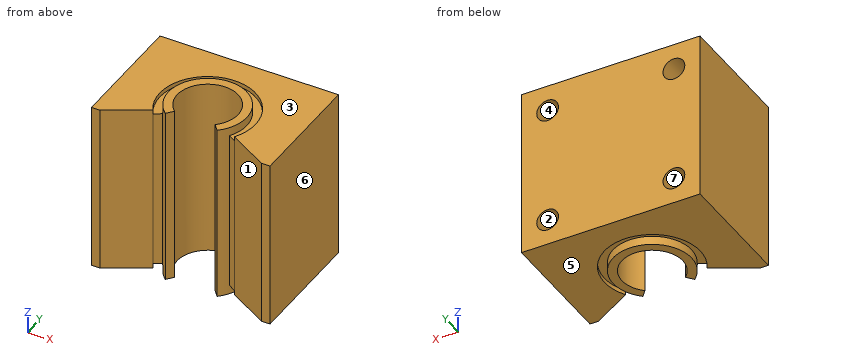
from build123d import *

# Parameters (mm, degrees)
BOSS_EXTRUDE1_DEPTH                  = 39
BOSS_EXTRUDE3_START                  = 1
BOSS_EXTRUDE3_DEPTH                  = 37
BOSS_EXTRUDE4_START                  = -1
BOSS_EXTRUDE4_DEPTH                  = 41
SKETCH4_R                            = 2.5
CUT_EXTRUDE1_DEPTH                   = 10
TAP_DRILL_FOR_M5X0_8_TAP1_AT_2_COUNT = 2
TAP_DRILL_FOR_M5X0_8_TAP1_AT_2_PITCH = 27
TAP_DRILL_FOR_M5X0_8_TAP1_AT_3_COUNT = 2
TAP_DRILL_FOR_M5X0_8_TAP1_AT_3_PITCH = 39.623223611
TAP_DRILL_FOR_M5X0_8_TAP1_AT_4_COUNT = 2
TAP_DRILL_FOR_M5X0_8_TAP1_AT_4_PITCH = 28.999998701


with BuildPart() as part:
    # Sketch1 → Boss-Extrude1 (new body)
    with BuildSketch(Plane.XY):
        with BuildLine():
            Line((-20.5, 14), (20.5, 14))
            Line((20.5, 14), (20.5, -14))
            Line((20.5, -14), (18.5, -14))
            Line((18.5, -14), (9.385134519, -8.737529961))
            ThreePointArc((9.385134519, -8.737529961), (0, 8), (-9.385134519, -8.737529961))
            Line((-9.385134519, -8.737529961), (-18.5, -14))
            Line((-18.5, -14), (-20.5, -14))
            Line((-20.5, -14), (-20.5, 14))
        make_face()
    extrude(amount=BOSS_EXTRUDE1_DEPTH)



with BuildPart() as body_2:
    # Sketch2 → Boss-Extrude3 (new body)
    with BuildSketch(Plane.XY.offset(BOSS_EXTRUDE3_START)):
        with BuildLine():
            Line((-9.385134519, -8.737529961), (-7.678746425, -7.694342695))
            ThreePointArc((-7.678746425, -7.694342695), (0, 6), (7.678746425, -7.694342695))
            Line((7.678746425, -7.694342695), (9.385134519, -8.737529961))
            ThreePointArc((9.385134519, -8.737529961), (0, 8), (-9.385134519, -8.737529961))
        make_face()
    extrude(amount=BOSS_EXTRUDE3_DEPTH)


with BuildPart() as part_1:
    add(part.part)

    add(body_2.part)  # Boss-Extrude4 merges body 2
    # Sketch3 → Boss-Extrude4 (add)
    with BuildSketch(Plane.XY.offset(BOSS_EXTRUDE4_START)):
        with BuildLine():
            Line((-5.9419479, -9.759678628), (-4.655936286, -8.227069666))
            ThreePointArc((-4.655936286, -8.227069666), (0, 4), (4.655936286, -8.227069666))
            Line((4.655936286, -8.227069666), (5.9419479, -9.759678628))
            ThreePointArc((5.9419479, -9.759678628), (0, 6), (-5.9419479, -9.759678628))
        make_face()
    extrude(amount=BOSS_EXTRUDE4_DEPTH)

    # Sketch4 → Cut-Extrude1 (cut)
    with BuildSketch(Plane(origin=(0, 14, 0), x_dir=(1, 0, 0), z_dir=(0, 1, 0))):
        with Locations(Location((-14.5, -6, 0), (0, 0, 270))):
            Circle(SKETCH4_R)
        with Locations(Location((14.499998701, -6, 0), (0, 0, 270))):
            Circle(SKETCH4_R)
        with Locations(Location((14.5, -33, 0), (0, 0, 270))):
            Circle(SKETCH4_R)
        with Locations(Location((-14.499998701, -33, 0), (0, 0, 270))):
            Circle(SKETCH4_R)
    extrude(amount=-CUT_EXTRUDE1_DEPTH, mode=Mode.SUBTRACT)

    # Sketch8 → Tap Drill for M5x0.8 Tap1 (revolve, cut)
    with BuildSketch(Plane(origin=(-14.499998701, 4, 33), x_dir=(0, 0, 1), z_dir=(1, 0, 0))):
        Polygon((0, 0), (0, 1.3118073), (2.1, 0.05), (2.1, 0.025), (2.125, 0), align=None)
    tap_drill_for_m5x0_8_tap1 = revolve(axis=Axis((-14.499998701, 10.35, 33), (0, -1, 0)), mode=Mode.SUBTRACT)

    # Tap Drill for M5x0.8 Tap1 at 2: Tap Drill for M5x0.8 Tap1 ×2
    with Locations(*[(0, 0, -i * TAP_DRILL_FOR_M5X0_8_TAP1_AT_2_PITCH) for i in range(1, TAP_DRILL_FOR_M5X0_8_TAP1_AT_2_COUNT)]):
        add(tap_drill_for_m5x0_8_tap1, mode=Mode.SUBTRACT)

    # Tap Drill for M5x0.8 Tap1 at 3: Tap Drill for M5x0.8 Tap1 ×2
    with Locations(*[Vector(0.7318939439938763, 0, -0.6814185606109426) * (i * TAP_DRILL_FOR_M5X0_8_TAP1_AT_3_PITCH) for i in range(1, TAP_DRILL_FOR_M5X0_8_TAP1_AT_3_COUNT)]):
        add(tap_drill_for_m5x0_8_tap1, mode=Mode.SUBTRACT)

    # Tap Drill for M5x0.8 Tap1 at 4: Tap Drill for M5x0.8 Tap1 ×2
    with Locations(*[(i * TAP_DRILL_FOR_M5X0_8_TAP1_AT_4_PITCH, 0, 0) for i in range(1, TAP_DRILL_FOR_M5X0_8_TAP1_AT_4_COUNT)]):
        add(tap_drill_for_m5x0_8_tap1, mode=Mode.SUBTRACT)


solid = part_1.part
The listing builds one solid part. Answer for the finished solid, in the listing's coordinates (mm). Face numbers are marked on the shaded views. A direction names the side the tool comes from. Coordinates: 2 decimals unless noted, no trailing zeros. Loops run counter-clockwise (first coordinate to the right, second up) from the corner with the lowest first, then second, coordinate; pieces in that order, holes last. Notation, with made-up numbers: (-2, 58) -> (32, 58) arc R29 cw to (32, 78) -> close; hole circle Ø11 at (27.5, 81). An arc over 180 degrees is marked (long way). Write item = value, one per line. Start each with the question number.
1) The mould has two halves that part along Z. Classify the marked faces 4, 5, 6 and 7: released by +Z, released by -Z, zero draft, split by the parting line, or undercut.
2) Straight lines are drawn through the part: line 1 (X direction, y = 4.05, z = 6); line 2 (X direction, y = 8, z = 31); line 3 (X direction, y = -2.75, z = 35). For each, find the intervals that lie inside material, in ascending order. Write a range as from..to.
3) A cutting plane is placed at A-A (y = -3). Give the vertices of the cut face in (x, z).
4) A cutting plane is placed at D-D (y = -12). Give the vertices of the cut face in (x, z), then the cut area to 3 significant figures.
5) A cutting plane is placed at B-B (x = 0). Give the vertices of the cut face in (y, z).
6) A cutting plane is placed at C-C (z = 22). Give the vertices of the cut face in (x, y).
7) Given pin 1 Ø4 at (x, z) = (4.5, 16.5) entering from -Y; pin 2 Ø2.5 at (x, z) = (-15.5, 33) entering from +Y; pin 3 Ø4.5 at (x, z) = (-14.5, 6) entering from -Y; pin 4 Ø8.5 at (x, y) = (0, -3) entering from +Z, each flat-ended and moving along its own axis, determine where each tip first touches the part or whether it passes through.
8) A tool of negligible diameter and unlimited length cuts with its end or side. For the marked faces 1, 2 and 3, from which of +Z, -Z, +X, -X, +Y, -Y can it reach the whole face along a straight path? Write none if from no direction.
Responses:
q1.face_4 = undercut
q1.face_5 = released by -Z
q1.face_6 = zero draft
q1.face_7 = undercut
q2.line_1 = -20.5..-17, -12..12, 17..20.5
q2.line_2 = -20.5..-16, -13..13, 16..20.5
q2.line_3 = -20.5..-7, 7..20.5
q3.outline = (-20.5, 0) -> (-11, 0) -> (-11, 1) -> (-9, 1) -> (-9, -1) -> (-7, -1) -> (-7, 40) -> (-9, 40) -> (-9, 38) -> (-11, 38) -> (-11, 39) -> (-20.5, 39) -> close; (7, -1) -> (9, -1) -> (9, 1) -> (11, 1) -> (11, 0) -> (20.5, 0) -> (20.5, 39) -> (11, 39) -> (11, 38) -> (9, 38) -> (9, 40) -> (7, 40) -> close
q4.outline = (-20.5, 0) -> (-15.04, 0) -> (-15.04, 39) -> (-20.5, 39) -> close; (15.04, 0) -> (20.5, 0) -> (20.5, 39) -> (15.04, 39) -> close
q4.area = 426 mm²
q5.outline = (4, -1) -> (6, -1) -> (6, 1) -> (8, 1) -> (8, 0) -> (14, 0) -> (14, 39) -> (8, 39) -> (8, 38) -> (6, 38) -> (6, 40) -> (4, 40) -> close
q6.outline = (-20.5, -14) -> (-18.5, -14) -> (-9.39, -8.74) -> (-7.68, -7.69) arc R9 ccw to (-5.94, -9.76) -> (-4.66, -8.23) arc R7 cw (long way) to (4.66, -8.23) -> (5.94, -9.76) arc R9 ccw to (7.68, -7.69) -> (9.39, -8.74) -> (18.5, -14) -> (20.5, -14) -> (20.5, 14) -> (-20.5, 14) -> close
q7.pin_1 = -9.76
q7.pin_2 = 4
q7.pin_3 = -12.99
q7.pin_4 = through
q8.face_1 = +Z, -Z, -Y
q8.face_2 = +Y
q8.face_3 = +Z, +Y
